Geometry check sheet. Reference: the model listing, model coordinates, mm. Face numbers are marked on the shaded views. A direction names the side the tool comes from. Round coordinates to 2 decimals unless told otherwise and drop trailing zeros. Write each loop counter-clockwise with the first axis right and the second up, starting at its lowest first coordinate (ties: lowest second). Pieces come first, ordered by that corner, then holes.
Item 1: Depth check by flat-ended pin: P1, Ø1, axis at x = 25, z = -3.5, coming from the -Y side; P2, Ø1.6, axis at x = 18.5, y = 0.5, coming from the +Z side. Enter the tip coordinate at first touch or a pass-through.
Item 2: Access from +Z, -Z, +X, -X, +Y, -Y to the whole of each face (thin tool, end or side, straight path). Record for the marked faces 1 and 2.
Item 3: Cross-section at C-C (z = -24). Enter the section's corners in (x, y).
Item 4: Cross-section at A-A (x = 0). Enter the section's corners in (y, z), then the cut area to 3 significant figures.
Item 5: Scan lines: probe 1 along Y at (x, z) = (-8, -18); probe 2 along X at (y, z) = (0.25, -20); probe 3 along X at (y, z) = (-2.5, -2). Record each from-to range of solid material in increasing order.
Item 6: Cross-section at D-D (x = -21.5). Enter the section's corners in (y, z), then the cut area to 3 significant figures.
Item 7: Cross-section at B-B (y = -4.75). Enter the section's corners in (x, z).
from build123d import *

# Parameters (mm, degrees)
BOSS_EXTRUDE1_DEPTH = 1
SKETCH3_R           = 2.75
BOSS_EXTRUDE2_DEPTH = 7
FILLET1_R           = 1


with BuildPart() as part:
    # Sketch1 → Boss-Extrude1 (new body)
    with BuildSketch(Plane(origin=(0, 0, 0), x_dir=(1, 0, 0), z_dir=(0, 1, 0))):
        with BuildLine():
            Line((-37.5, 0), (37.5, 0))
            ThreePointArc((37.5, 0), (0, 37.5), (-37.5, 0))
        make_face()
    extrude(amount=BOSS_EXTRUDE1_DEPTH)

    # Sketch3 → Boss-Extrude2 (add)
    with BuildSketch(Plane(origin=(0, 1, 0), x_dir=(1, 0, 0), z_dir=(0, 1, 0))):
        with Locations(Location((0, 0, 0), (0, 0, 270))):
            Circle(SKETCH3_R)
    extrude(amount=-BOSS_EXTRUDE2_DEPTH)

    # Fillet1
    fillet1_edges = [part.edges().sort_by_distance(p)[0] for p in [
        (0, 0, -2.75),
    ]]
    fillet(fillet1_edges, radius=FILLET1_R)


solid = part.part
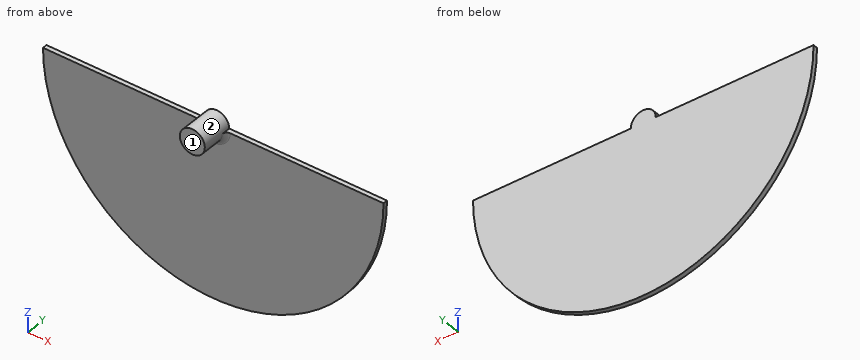
Resolved:
1. P1: stops at y = 0
1. P2: stops at z = 0
2. face 1: +Z, -Z, +X, -X, -Y
2. face 2: -Y
3. outline: (-28.81, 0) - (28.81, 0) - (28.81, 1) - (-28.81, 1) - close
4. outline: (-6, -2.75) - (-1, -2.75) arc R1 cw to (0, -3.75) - (0, -37.5) - (1, -37.5) - (1, 2.75) - (-6, 2.75) - close
4. area: 73.5 mm2
5. probe 1: y = 0 to 1
5. probe 2: x = -31.72 to 31.72
5. probe 3: x = -1.89 to 1.89
6. outline: (0, -30.72) - (1, -30.72) - (1, 0) - (0, 0) - close
6. area: 30.7 mm2
7. outline: circle Ø5.5 at (0, 0)
